Design review of the part built by this model. Coordinates are the model's own, in mm. A direction names the side the tool comes from. Round coordinates to 2 decimals unless told otherwise and drop trailing zeros. Order: outer loops, then holes, each group sorted by start corner. A loop starts at its lowest first (then second) coordinate and runs counter-clockwise, first axis right, second up. Notation, with made-up numbers: (41.25, 89.25) - (98.25, 89.25) arc R17 ccw to (98.25, 101.25) - close; hole circle Ø1 at (10, 9). An arc over 180 degrees is marked (long way). Write item = value, one per line.
from build123d import *

# Parameters (mm, degrees)
F0_W     = 19.05
F0_H     = 38.1
F1_DEPTH = 57.15
F2_R     = 12.7
F3_DEPTH = 12.7
F5_D     = 3.175
F5_DEPTH = 6.35
F5_TIP   = 0.9538662327


with BuildPart() as f1:
    # F0 (on Right) → F1 (new body, symmetric)
    with BuildSketch(Plane.YZ):
        with Locations((9.525, 19.05)):
            Rectangle(F0_W, F0_H)
    extrude(amount=F1_DEPTH, both=True)

    # F2 (on face) → F3 (cut)
    with BuildSketch(Plane.XZ):
        with Locations((0, 15.875)):
            Circle(F2_R)
    extrude(amount=-F3_DEPTH, mode=Mode.SUBTRACT)

    # F5
    with Locations(Plane.XY.offset(38.1)):
        with Locations((0, 14.2748), (-47.625, 14.2748), (-14.2875, 6.025908029), (-23.8125, 6.025908029), (23.8125, 6.025908029), (-33.3375, 6.025908029), (28.575, 14.2748), (4.7625, 6.025908029), (-4.7625, 6.025908029), (-19.05, 14.2748), (14.2875, 6.025908029), (9.525, 14.2748), (19.05, 14.2748), (42.8625, 6.025908029), (33.3375, 6.025908029), (47.625, 14.2748), (-42.8625, 6.025908029), (38.1, 14.2748), (-28.575, 14.2748), (-9.525, 14.2748), (-38.1, 14.2748)):
            Hole(F5_D / 2, depth=F5_DEPTH)
            with Locations((0, 0, -(F5_DEPTH + F5_TIP / 2))):  # 118° drill point
                Cone(0, F5_D / 2, F5_TIP, mode=Mode.SUBTRACT)


solid = f1.part
Item 1: Insertion check: P1, Ø6, axis at x = 1, z = 11, coming from the -Y side; P2, Ø3, axis at x = -47.62, y = 14.27, coming from the +Z side; P3, Ø1.9, axis at x = 14.29, y = 6.03, coming from the +Z side; P4, Ø5, axis at x = -14.29, y = 6.03, coming from the -Z side. Each pin has a flat end and moves straight along its axis. Give the tip position at first contact, or say it passes through.
Data:
P1 = 12.7
P2 = 31.7
P3 = 31.37
P4 = 0
Item 2: Take a section at A-A, the plane y = 8.75. State the section outline as (x, z) points (3 decimals), and give its area (3 significant figures).
Data:
outline = (-57.15, 0) - (57.15, 0) - (57.15, 38.1) - (-57.15, 38.1) - close; hole circle Ø25.4 at (0, 15.875)
area = 3,850 mm2
Item 3: The part is to be moulded in two halves that separate along X. For faces 1 (the face through (57.15, 9, 19)), 2 (the face through (14, 0, 19)), 3 (the face through (-18.706, 12.725, 34.881)), say which applies: +X half, -X half, draft (parallel to the pull), parting line (faces both ways), or undercut.
Data:
face_1 = +X half
face_2 = draft
face_3 = undercut
Item 4: Take a section at B-B, the plane z = 21.5. State the section outline as (x, y) points.
Data:
outline = (-57.15, 0) - (-11.39, 0) - (-11.39, 12.7) - (11.39, 12.7) - (11.39, 0) - (57.15, 0) - (57.15, 19.05) - (-57.15, 19.05) - close
Item 5: Take a section at C-C, the plane z = 26. State the section outline as (x, y) points, and give its area (3 significant figures).
Data:
outline = (-57.15, 0) - (-7.67, 0) - (-7.67, 12.7) - (7.67, 12.7) - (7.67, 0) - (57.15, 0) - (57.15, 19.05) - (-57.15, 19.05) - close
area = 1,980 mm2
Item 6: For line 1 along Y through (x, z) = (0, 36.75); line 2 along X through (y, z) = (8, 16.5); line 3 along Y through (x, z) = (-7.5, 22), list the stretches that pass through material, from the lowest coordinate up. Write a range as [from, to].
Data:
line_1 = [0, 12.69], [15.86, 19.05]
line_2 = [-57.15, -12.68], [12.68, 57.15]
line_3 = [12.7, 19.05]
Item 7: For faces 4 (the face through (-38.833, 12.866, 34.881)), 5 (the face through (1, 19.05, 19)), list the 3-axis set-ups (+Z, -Z, +X, -X, +Y, -Y) from which the entire face can be reached by the end or side of a thin tool; tool diameter is ignored.
Data:
face_4 = +Z
face_5 = +Z, -Z, +X, -X, +Y
